The figure shows three views and two pictorial views of one solid part (mm, origin at its lowest corner). Answer the questions. A direction names the side the tool comes from. Give positions to 0.01 mm unless a question says otherwise; leave off trailing zeros. Write each loop counter-clockwise with the first axis right and the second up, starting at its lowest first coordinate (ties: lowest second). Pieces come first, ordered by that corner, then holes. Notation, with made-up numbers: (84, 15) -> (107, 15) arc R30 ccw to (107, 37) -> close; hole circle Ø11 at (51.5, 75). An arc over 180 degrees is marked (long way). Use a Markdown table: item, result.
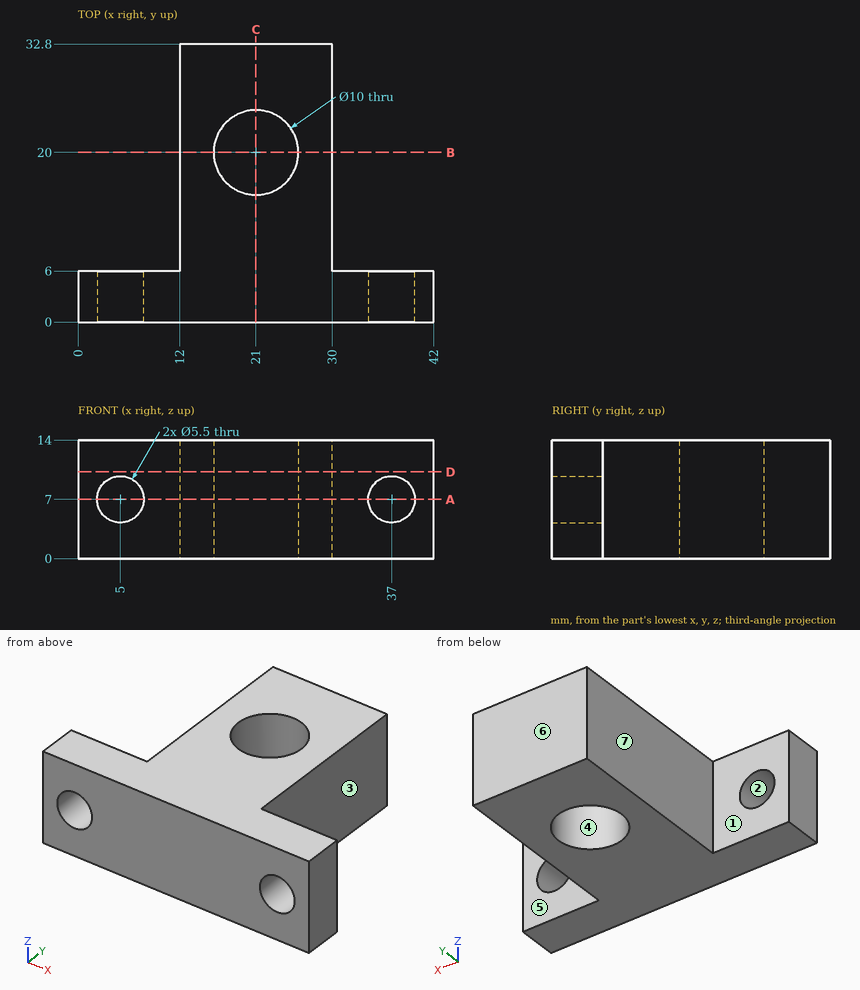
Item 1: A cutting plane is placed at A-A (z = 7). Give the vertices of the cut face in (x, y).
Return value:
| item | result |
|---|---|
| outline | (0, 0) -> (2.25, 0) -> (2.25, 6) -> (0, 6) -> close; (7.75, 0) -> (34.25, 0) -> (34.25, 6) -> (30, 6) -> (30, 32.8) -> (12, 32.8) -> (12, 6) -> (7.75, 6) -> close; (39.75, 0) -> (42, 0) -> (42, 6) -> (39.75, 6) -> close; hole circle Ø10 at (21, 20) |
Item 2: A tool of negligible diameter and unlimited length cuts with its end or side. For the marked faces 5, 6 and 7, from which of +Z, -Z, +X, -X, +Y, -Y can it reach the whole face along a straight path? Write none if from no direction.
Return value:
| item | result |
|---|---|
| face 5 | +Z, -Z, +X, +Y |
| face 6 | +Z, -Z, +X, -X, +Y |
| face 7 | +Z, -Z, -X, +Y |
Item 3: Each of these flat-tipped pins is pushed along its axis until it touches: P1, Ø7, axis at y = 22.5, z = 9.5, coming from the -X side; P2, Ø3.5, axis at x = 34.5, z = 9.5, coming from the +Y side; P3, Ø8, axis at x = 21, y = 20, coming from the +Z side; P4, Ø2, axis at y = 20.5, z = 9.5, coming from the +X side. Where does it stop, or does it pass through?
Return value:
| item | result |
|---|---|
| P1 | x = 12 |
| P2 | y = 6 |
| P3 | through |
| P4 | x = 30 |
Item 4: A cutting plane is placed at C-C (x = 21). Give the vertices of the cut face in (y, z).
Return value:
| item | result |
|---|---|
| outline | (0, 0) -> (15, 0) -> (15, 14) -> (0, 14) -> close; (25, 0) -> (32.8, 0) -> (32.8, 14) -> (25, 14) -> close |
Item 5: A cutting plane is placed at B-B (y = 20). Give the vertices of the cut face in (x, z).
Return value:
| item | result |
|---|---|
| outline | (12, 0) -> (16, 0) -> (16, 14) -> (12, 14) -> close; (26, 0) -> (30, 0) -> (30, 14) -> (26, 14) -> close |
Item 6: A cutting plane is placed at D-D (z = 10.25). Give the vertices of the cut face in (x, y).
Return value:
| item | result |
|---|---|
| outline | (0, 0) -> (42, 0) -> (42, 6) -> (30, 6) -> (30, 32.8) -> (12, 32.8) -> (12, 6) -> (0, 6) -> close; hole circle Ø10 at (21, 20) |
Item 7: Straight lines are drawn through the part: line 1 along Z through (x, y) = (5, 4.25); line 2 along Y through (x, z) = (33.5, 1.75); line 3 along Y through (x, z) = (21, 4.5). For each, find the intervals that lie inside material, in ascending order. Write a range as [from, to].
Return value:
| item | result |
|---|---|
| line 1 | [0, 4.25], [9.75, 14] |
| line 2 | [0, 6] |
| line 3 | [0, 15], [25, 32.8] |
Item 8: For a pull along X with two mould halves and no side action, classify the marked faces 1, 2, 3 and 4 as +X half, -X half, draft (parallel to the pull), parting line (faces both ways), or undercut.
Return value:
| item | result |
|---|---|
| face 1 | draft |
| face 2 | undercut |
| face 3 | +X half |
| face 4 | undercut |
